Geometry: final body of the model. Coordinates: model frame, mm. Face numbers are marked on the shaded views. A direction names the side the tool comes from. Give positions to 0.01 mm unless a question says otherwise; leave off trailing zeros. Write each loop counter-clockwise with the first axis right and the second up, starting at its lowest first coordinate (ties: lowest second). Pieces come first, ordered by that corner, then holes.
from build123d import *

# Parameters (mm, degrees)
BOSS_EXTRUDE1_DEPTH = 8
SKETCH2_R           = 180
BOSS_EXTRUDE2_DEPTH = 1
CUT_EXTRUDE1_REACH  = 10
SKETCH3_R           = 2


with BuildPart() as part:
    # Sketch1 → Boss-Extrude1 (new body)
    with BuildSketch(Plane.XY):
        Polygon((5, 230), (5, 180), (-5, 180), (-5, 230), (-7, 230), (-157.684812205, 167.584307141), (-159.099025767, 166.170093579), (-123.743686708, 130.814754519), (-130.81475452, 123.743686708), (-166.170093579, 159.099025767), (-167.584307141, 157.684812205), (-230, 7), (-230, 5), (-180, 5), (-180, -5), (-230, -5), (-230, -7), (-167.584307141, -157.684812205), (-166.170093579, -159.099025767), (-130.81475452, -123.743686708), (-123.743686708, -130.81475452), (-159.099025767, -166.170093579), (-157.684812205, -167.584307141), (-7, -230), (-5, -230), (-5, -180), (5, -180), (5, -230), (7, -230), (157.684812205, -167.584307141), (159.099025767, -166.170093579), (123.743686708, -130.814754519), (130.81475452, -123.743686708), (166.170093579, -159.099025767), (167.584307141, -157.684812205), (230, -7), (230, -5), (180, -5), (180, 5), (230, 5), (230, 7), (167.584307141, 157.684812205), (166.170093579, 159.099025767), (130.81475452, 123.743686708), (123.743686708, 130.81475452), (159.099025767, 166.170093579), (157.684812205, 167.584307141), (7, 230), align=None)
    extrude(amount=BOSS_EXTRUDE1_DEPTH)

    # Sketch2 → Boss-Extrude2 (add)
    with BuildSketch(Plane.XY.offset(8)):
        Circle(SKETCH2_R)
    extrude(amount=BOSS_EXTRUDE2_DEPTH)

    # Sketch3 → Cut-Extrude1 (cut, up to next)
    with BuildSketch(Plane.XY.offset(8), mode=Mode.PRIVATE) as cut_extrude1_sk1:
        with Locations((107.397750993, 174.354514299)):
            Circle(SKETCH3_R)
    cut_extrude1_tool1 = extrude(cut_extrude1_sk1.sketch, amount=-CUT_EXTRUDE1_REACH, mode=Mode.PRIVATE) & part.part
    add(cut_extrude1_tool1.solids().sort_by_distance((107.397751, 174.354514, 8))[0], mode=Mode.SUBTRACT)
    # Sketch3 → Cut-Extrude1 (cut, up to next)
    with BuildSketch(Plane.XY.offset(8), mode=Mode.PRIVATE) as cut_extrude1_sk2:
        with Locations((47.34558138, 199.228937402)):
            Circle(SKETCH3_R)
    cut_extrude1_tool2 = extrude(cut_extrude1_sk2.sketch, amount=-CUT_EXTRUDE1_REACH, mode=Mode.PRIVATE) & part.part
    add(cut_extrude1_tool2.solids().sort_by_distance((47.345581, 199.228937, 8))[0], mode=Mode.SUBTRACT)
    # Sketch3 → Cut-Extrude1 (cut, up to next)
    with BuildSketch(Plane.XY.offset(8), mode=Mode.PRIVATE) as cut_extrude1_sk3:
        with Locations((199.228937402, 47.34558138)):
            Circle(SKETCH3_R)
    cut_extrude1_tool3 = extrude(cut_extrude1_sk3.sketch, amount=-CUT_EXTRUDE1_REACH, mode=Mode.PRIVATE) & part.part
    add(cut_extrude1_tool3.solids().sort_by_distance((199.228937, 47.345581, 8))[0], mode=Mode.SUBTRACT)
    # Sketch3 → Cut-Extrude1 (cut, up to next)
    with BuildSketch(Plane.XY.offset(8), mode=Mode.PRIVATE) as cut_extrude1_sk4:
        with Locations((174.354514299, 107.397750993)):
            Circle(SKETCH3_R)
    cut_extrude1_tool4 = extrude(cut_extrude1_sk4.sketch, amount=-CUT_EXTRUDE1_REACH, mode=Mode.PRIVATE) & part.part
    add(cut_extrude1_tool4.solids().sort_by_distance((174.354514, 107.397751, 8))[0], mode=Mode.SUBTRACT)
    # Sketch3 → Cut-Extrude1 (cut, up to next)
    with BuildSketch(Plane.XY.offset(8), mode=Mode.PRIVATE) as cut_extrude1_sk5:
        with Locations((174.354514299, -107.397750993)):
            Circle(SKETCH3_R)
    cut_extrude1_tool5 = extrude(cut_extrude1_sk5.sketch, amount=-CUT_EXTRUDE1_REACH, mode=Mode.PRIVATE) & part.part
    add(cut_extrude1_tool5.solids().sort_by_distance((174.354514, -107.397751, 8))[0], mode=Mode.SUBTRACT)
    # Sketch3 → Cut-Extrude1 (cut, up to next)
    with BuildSketch(Plane.XY.offset(8), mode=Mode.PRIVATE) as cut_extrude1_sk6:
        with Locations((199.228937402, -47.34558138)):
            Circle(SKETCH3_R)
    cut_extrude1_tool6 = extrude(cut_extrude1_sk6.sketch, amount=-CUT_EXTRUDE1_REACH, mode=Mode.PRIVATE) & part.part
    add(cut_extrude1_tool6.solids().sort_by_distance((199.228937, -47.345581, 8))[0], mode=Mode.SUBTRACT)
    # Sketch3 → Cut-Extrude1 (cut, up to next)
    with BuildSketch(Plane.XY.offset(8), mode=Mode.PRIVATE) as cut_extrude1_sk7:
        with Locations((47.34558138, -199.228937402)):
            Circle(SKETCH3_R)
    cut_extrude1_tool7 = extrude(cut_extrude1_sk7.sketch, amount=-CUT_EXTRUDE1_REACH, mode=Mode.PRIVATE) & part.part
    add(cut_extrude1_tool7.solids().sort_by_distance((47.345581, -199.228937, 8))[0], mode=Mode.SUBTRACT)
    # Sketch3 → Cut-Extrude1 (cut, up to next)
    with BuildSketch(Plane.XY.offset(8), mode=Mode.PRIVATE) as cut_extrude1_sk8:
        with Locations((107.397750993, -174.354514299)):
            Circle(SKETCH3_R)
    cut_extrude1_tool8 = extrude(cut_extrude1_sk8.sketch, amount=-CUT_EXTRUDE1_REACH, mode=Mode.PRIVATE) & part.part
    add(cut_extrude1_tool8.solids().sort_by_distance((107.397751, -174.354514, 8))[0], mode=Mode.SUBTRACT)
    # Sketch3 → Cut-Extrude1 (cut, up to next)
    with BuildSketch(Plane.XY.offset(8), mode=Mode.PRIVATE) as cut_extrude1_sk9:
        with Locations((-107.397750993, -174.354514299)):
            Circle(SKETCH3_R)
    cut_extrude1_tool9 = extrude(cut_extrude1_sk9.sketch, amount=-CUT_EXTRUDE1_REACH, mode=Mode.PRIVATE) & part.part
    add(cut_extrude1_tool9.solids().sort_by_distance((-107.397751, -174.354514, 8))[0], mode=Mode.SUBTRACT)
    # Sketch3 → Cut-Extrude1 (cut, up to next)
    with BuildSketch(Plane.XY.offset(8), mode=Mode.PRIVATE) as cut_extrude1_sk10:
        with Locations((-47.34558138, -199.228937402)):
            Circle(SKETCH3_R)
    cut_extrude1_tool10 = extrude(cut_extrude1_sk10.sketch, amount=-CUT_EXTRUDE1_REACH, mode=Mode.PRIVATE) & part.part
    add(cut_extrude1_tool10.solids().sort_by_distance((-47.345581, -199.228937, 8))[0], mode=Mode.SUBTRACT)
    # Sketch3 → Cut-Extrude1 (cut, up to next)
    with BuildSketch(Plane.XY.offset(8), mode=Mode.PRIVATE) as cut_extrude1_sk11:
        with Locations((-199.228937402, -47.34558138)):
            Circle(SKETCH3_R)
    cut_extrude1_tool11 = extrude(cut_extrude1_sk11.sketch, amount=-CUT_EXTRUDE1_REACH, mode=Mode.PRIVATE) & part.part
    add(cut_extrude1_tool11.solids().sort_by_distance((-199.228937, -47.345581, 8))[0], mode=Mode.SUBTRACT)
    # Sketch3 → Cut-Extrude1 (cut, up to next)
    with BuildSketch(Plane.XY.offset(8), mode=Mode.PRIVATE) as cut_extrude1_sk12:
        with Locations((-174.354514299, -107.397750993)):
            Circle(SKETCH3_R)
    cut_extrude1_tool12 = extrude(cut_extrude1_sk12.sketch, amount=-CUT_EXTRUDE1_REACH, mode=Mode.PRIVATE) & part.part
    add(cut_extrude1_tool12.solids().sort_by_distance((-174.354514, -107.397751, 8))[0], mode=Mode.SUBTRACT)
    # Sketch3 → Cut-Extrude1 (cut, up to next)
    with BuildSketch(Plane.XY.offset(8), mode=Mode.PRIVATE) as cut_extrude1_sk13:
        with Locations((-174.354514299, 107.397750993)):
            Circle(SKETCH3_R)
    cut_extrude1_tool13 = extrude(cut_extrude1_sk13.sketch, amount=-CUT_EXTRUDE1_REACH, mode=Mode.PRIVATE) & part.part
    add(cut_extrude1_tool13.solids().sort_by_distance((-174.354514, 107.397751, 8))[0], mode=Mode.SUBTRACT)
    # Sketch3 → Cut-Extrude1 (cut, up to next)
    with BuildSketch(Plane.XY.offset(8), mode=Mode.PRIVATE) as cut_extrude1_sk14:
        with Locations((-199.228937402, 47.34558138)):
            Circle(SKETCH3_R)
    cut_extrude1_tool14 = extrude(cut_extrude1_sk14.sketch, amount=-CUT_EXTRUDE1_REACH, mode=Mode.PRIVATE) & part.part
    add(cut_extrude1_tool14.solids().sort_by_distance((-199.228937, 47.345581, 8))[0], mode=Mode.SUBTRACT)
    # Sketch3 → Cut-Extrude1 (cut, up to next)
    with BuildSketch(Plane.XY.offset(8), mode=Mode.PRIVATE) as cut_extrude1_sk15:
        with Locations((-47.34558138, 199.228937402)):
            Circle(SKETCH3_R)
    cut_extrude1_tool15 = extrude(cut_extrude1_sk15.sketch, amount=-CUT_EXTRUDE1_REACH, mode=Mode.PRIVATE) & part.part
    add(cut_extrude1_tool15.solids().sort_by_distance((-47.345581, 199.228937, 8))[0], mode=Mode.SUBTRACT)
    # Sketch3 → Cut-Extrude1 (cut, up to next)
    with BuildSketch(Plane.XY.offset(8), mode=Mode.PRIVATE) as cut_extrude1_sk16:
        with Locations((-107.397750993, 174.354514299)):
            Circle(SKETCH3_R)
    cut_extrude1_tool16 = extrude(cut_extrude1_sk16.sketch, amount=-CUT_EXTRUDE1_REACH, mode=Mode.PRIVATE) & part.part
    add(cut_extrude1_tool16.solids().sort_by_distance((-107.397751, 174.354514, 8))[0], mode=Mode.SUBTRACT)


solid = part.part
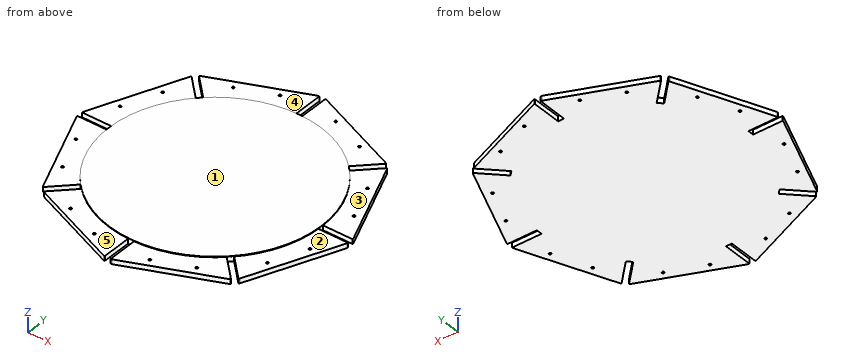
Q1. Section B-B on x = 26. Output: boundary loops of the cut face in (y, z), plus the area to 3 significant figures.
Filled sheet:
outline: (-222.13, 0) - (222.13, 0) - (222.13, 8) - (178.11, 8) - (178.11, 9) - (-178.11, 9) - (-178.11, 8) - (-222.13, 8) - close
area: 3,910 mm2
Q2. Section C-C on z = 2.25. Count the separate pieces of the cut face and the enclosed holes in it, plus the area to 3 significant figures.
Filled sheet:
separate pieces: 1
enclosed holes: 16
area: 149,000 mm2
Q3. Pin query (flat end, axial travel): P1, Ø2, axis at y = -121.5, z = 8, coming from the +X side; P2, Ø5, axis at x = 14.5, z = 4.5, coming from the +Y side; P3, Ø5, axis at x = -121.5, y = -87.5, coming from the -Z side; P4, Ø2.5, axis at y = 208, z = 5.5, coming from the -X side. Return the tip coordinate at first contact, or that it passes through.
Filled sheet:
P1: stops at x = 182.99
P2: stops at y = 227.93
P3: stops at z = 0
P4: stops at x = -63.13
Q4. Access query for the marked faces 1, 2, 3, 4 and 5. Directions: +Z, -Z, +X, -X, +Y, -Y. A direction counts if a zero-diameter tool reaches every point of the face in a straight line with its end or side. Return the directions, or none.
Filled sheet:
face 1: +Z, +X, -X, +Y, -Y
face 2: +Z, +X, -Y
face 3: +Z, +X, +Y
face 4: +Z, -X, +Y
face 5: +Z, -X, -Y
Q5. Ray query, line 1 along X through (y, z) = (140.5, 4.25); line 2 along Z through (x, y) = (11, -188); line 3 along Y through (x, z) = (-137, 5). Return the intervals inside material, ascending.
Filled sheet:
line 1: x = -174.7 to -147.57, -133.43 to 133.43, 147.57 to 174.7
line 2: z = 0 to 8
line 3: y = -176.15 to -144.07, -129.93 to 129.93, 144.07 to 176.15
Q6. Section A-A on y = 72. Output: boundary loops of the cut face in (x, z).
Filled sheet:
outline: (-203.08, 0) - (203.08, 0) - (203.08, 8) - (164.97, 8) - (164.97, 9) - (-164.97, 9) - (-164.97, 8) - (-203.08, 8) - close
